from build123d import *

# Parameters (mm, degrees)
SKETCH2_R          = 1.6002
CUT_EXTRUDE1_DEPTH = 12.7
SKETCH3_R          = 1.1811
CUT_EXTRUDE2_DEPTH = 12.7


with BuildPart() as part:
    # Sketch1 → Revolve1 (revolve)
    with BuildSketch(Plane.XY, mode=Mode.PRIVATE) as revolve1_sk:
        with BuildLine():
            Line((0, 83.34375), (-6.35, 83.34375))
            Line((-6.35, 83.34375), (-6.35, 73.025))
            ThreePointArc((-6.35, 73.025), (-6.582483992, 72.463733992), (-7.14375, 72.23125))
            Line((-7.14375, 72.23125), (-9.5377, 72.23125))
            Line((-9.5377, 72.23125), (-9.5377, 61.9125))
            ThreePointArc((-9.5377, 61.9125), (-9.770183992, 61.351233992), (-10.33145, 61.11875))
            Line((-10.33145, 61.11875), (-12.7, 61.11875))
            Line((-12.7, 61.11875), (-12.7, 0))
            Line((-12.7, 0), (-12.7, -61.11875))
            Line((-12.7, -61.11875), (-10.30605, -61.11875))
            ThreePointArc((-10.30605, -61.11875), (-9.744783992, -61.351233992), (-9.5123, -61.9125))
            Line((-9.5123, -61.9125), (-9.5123, -105.56875))
            Line((-9.5123, -105.56875), (0, -105.56875))
            Line((0, -105.56875), (0, 83.34375))
        make_face()
    revolve(revolve1_sk.sketch.rotate(Axis((0, -122.193490481, 0), (0, 1, 0)), 270), axis=Axis((0, -122.193490481, 0), (0, 1, 0)))

    # Sketch2 → Cut-Extrude1 (cut)
    with BuildSketch(Plane(origin=(0, 83.34375, 0), x_dir=(1, 0, 0), z_dir=(0, 1, 0))):
        with Locations(Location((0, 0, 0), (0, 0, 270))):
            Circle(SKETCH2_R)
    extrude(amount=-CUT_EXTRUDE1_DEPTH, mode=Mode.SUBTRACT)

    # Sketch3 → Cut-Extrude2 (cut, symmetric)
    with BuildSketch(Plane(origin=(0, 0, 0), x_dir=(0, 0, -1), z_dir=(1, 0, 0))):
        with Locations((0, 78.58125)):
            Circle(SKETCH3_R)
    extrude(amount=CUT_EXTRUDE2_DEPTH, both=True, mode=Mode.SUBTRACT)


solid = part.part
Geometry: final body of the model. Coordinates: model frame, mm. A direction names the side the tool comes from. Round coordinates to 2 decimals unless told otherwise and drop trailing zeros. Loops run counter-clockwise (first coordinate to the right, second up) from the corner with the lowest first, then second, coordinate; pieces in that order, holes last.
Q1. Material intervals for L1, parallel to X at y = 76.5, z = 0; L2, parallel to Y at x = -4.5, z = 6.5; L3, parallel to Y at x = -3.7, z = 0, sorted ascending.
Q2. Section A-A on y = -24. Return loops of the section in (x, z), plus the area to 3 significant figures.
Q3. Pin query (flat end, axial travel): P1, Ø8, axis at y = -67.5, z = 8, coming from the +X side; P2, Ø1.9, axis at x = 0, z = 0, coming from the +Y side; P3, Ø2, axis at x = -6.5, y = -38, coming from the +Z side; P4, Ø12, axis at x = -6.5, z = 8.5, coming from the +Y side. Return the tip coordinate at first contact, or that it passes through.
Q4. Section B-B on y = 67.5. Return loops of the section in (x, z).
Q5. Pull-direction query (X, two-part tool) for faces 1 (the cylindrical face through (0.07, 77.08, -1.6)), 2 (the cylindrical face through (7.7, -0.9, 10.1)), 3 (the flat face through (-6.4, 72.231, 3.5)), 4 (the flat face through (0, 70.644, 0)); classes: released by +X, released by -X, zero draft, split by the parting line, or undercut.
Q6. Access query for faces 5 (the flat face through (1.3, 83.344, 1.3)), 6 (the cylindrical face through (9.31, 67, 2.07)), 7 (the flat face through (-10.41, -61.119, 1)). Directions: +Z, -Z, +X, -X, +Y, -Y. A direction counts if a zero-diameter tool reaches every point of the face in a straight line with its end or side. Return the directions, or none.
Evaluation:
1. L1: x = -6.35 to -1.6, 1.6 to 6.35
1. L2: y = -105.57 to 72.23
1. L3: y = -105.57 to 77.4, 79.76 to 83.34
2. outline: circle Ø25.4 at (0, 0)
2. area: 507 mm2
3. P1: stops at x = 8.63
3. P2: stops at y = 70.64
3. P3: stops at z = 11.45
3. P4: stops at y = 83.34
4. outline: circle Ø19.08 at (0, 0)
5. face 1: undercut
5. face 2: split by the parting line
5. face 3: zero draft
5. face 4: undercut
6. face 5: +Z, -Z, +X, -X, +Y
6. face 6: +Y
6. face 7: -Y
